Part print with two shaded views. Sizes in mm from the minimum x, y, z corner. Coordinates: 2 decimals unless noted, no trailing zeros. Order: outer loops, then holes, each group sorted by start corner. A loop starts at its lowest first (then second) coordinate and runs counter-clockwise, first axis right, second up. Notation, with made-up numbers: (-24, -28) - (-1, -28) arc R16 ccw to (-1, 3) - close; hole circle Ø10 at (52, 49.5). An arc over 180 degrees is marked (long way). One line per item, written item: value.
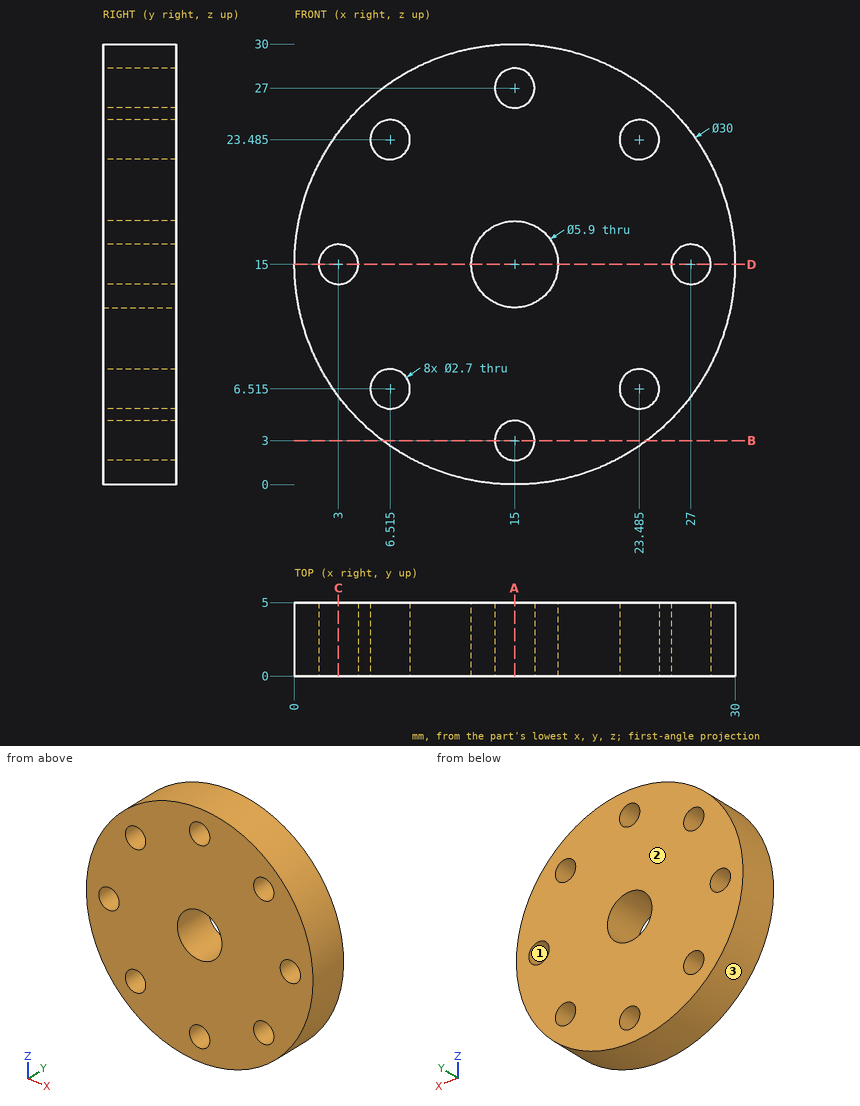
1. Band-saw the part on A-A, the plane x = 15. Give the cut face in (y, z).
Values found:
outline: (0, 0) - (5, 0) - (5, 1.65) - (0, 1.65) - close; (0, 4.35) - (5, 4.35) - (5, 12.05) - (0, 12.05) - close; (0, 17.95) - (5, 17.95) - (5, 25.65) - (0, 25.65) - close; (0, 28.35) - (5, 28.35) - (5, 30) - (0, 30) - close
2. Two-plate mould, pull along X, no slides. Class the marked faces 1, 2 and 3: pulls with the +X half, pulls with the -X half, needs draft (parallel to the pull), parting line crosses it, or undercut.
Values found:
face 1: undercut
face 2: needs draft
face 3: parting line crosses it
3. Band-saw the part on B-B, the plane z = 3. Give the cut face in (x, y), and give its area (3 significant figures).
Values found:
outline: (6, 0) - (13.65, 0) - (13.65, 5) - (6, 5) - close; (16.35, 0) - (24, 0) - (24, 5) - (16.35, 5) - close
area: 76.5 mm2
4. Probe line 1 along X through (y, z) = (3.3, 15); line 2 along Z through (x, y) = (14, 4.55) (1 decimal); line 3 along Z through (x, y) = (3.25, 3.8) (1 decimal). List the from-to ranges inside material, lowest first.
Values found:
line 1: x = 0 to 1.65, 4.35 to 12.05, 17.95 to 25.65, 28.35 to 30
line 2: z = 0 to 2.1, 3.9 to 12.2, 17.8 to 26.1, 27.9 to 30
line 3: z = 5.7 to 13.7, 16.3 to 24.3
5. Band-saw the part on D-D, the plane z = 15. Give the cut face in (x, y).
Values found:
outline: (0, 0) - (1.65, 0) - (1.65, 5) - (0, 5) - close; (4.35, 0) - (12.05, 0) - (12.05, 5) - (4.35, 5) - close; (17.95, 0) - (25.65, 0) - (25.65, 5) - (17.95, 5) - close; (28.35, 0) - (30, 0) - (30, 5) - (28.35, 5) - close
6. Band-saw the part on C-C, the plane x = 3. Give the cut face in (y, z), and give its area (3 significant figures).
Values found:
outline: (0, 6) - (5, 6) - (5, 13.65) - (0, 13.65) - close; (0, 16.35) - (5, 16.35) - (5, 24) - (0, 24) - close
area: 76.5 mm2
7. Flat gauge pins, fed straight in: P1, Ø2, axis at y = 3.5, z = 20, coming from the -X side; P2, Ø1, axis at x = 24, y = 2.5, coming from the +Z side. Where does each tip first touch, or does it go through?
Values found:
P1: stops at x = 0.54
P2: stops at z = 27.36
